Can you work these out from the model? Positions are in its coordinate system, mm. Face numbers are marked on the shaded views. A direction names the side the tool comes from. Round coordinates to 2 decimals unless told otherwise and drop trailing zeros. Loops run counter-clockwise (first coordinate to the right, second up) from the corner with the lowest first, then second, coordinate; pieces in that order, holes last. Notation, with made-up numbers: (64, 55.25) -> (84, 55.25) arc R9 ccw to (84, 61.25) -> close; hole circle Ø3 at (7, 1). An arc over 180 degrees is marked (long way). Use a Markdown table: item, result.
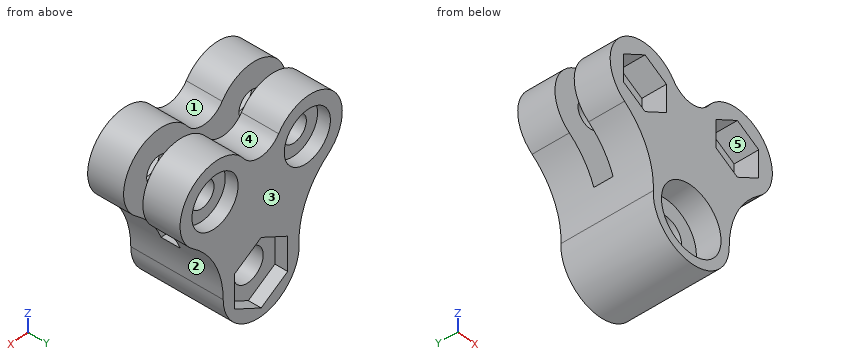
from build123d import *

# Parameters (mm, degrees)
SKETCH1_R           = 3.2639
SKETCH1_R_2         = 4.1021
BOSS_EXTRUDE1_DEPTH = 22.86
CUT_EXTRUDE1_DEPTH  = 4.7625
SKETCH3_R           = 8.1915
BOTTOM_CUTS_DEPTH   = 6.096
SKETCH4_R           = 6.35
TOP_CUTS_DEPTH      = 3.175


with BuildPart() as part:
    # Sketch1 → Boss-Extrude1 (new body)
    with BuildSketch(Plane(origin=(0, 0, 0), x_dir=(1, 0, 0), z_dir=(0, 1, 0))):
        with BuildLine():
            ThreePointArc((-10.440306098, 157.003610008), (-12.313301142, 147.763224627), (-18.350908637, 140.521668981))
            ThreePointArc((-18.350908637, 140.521668981), (-19.427506678, 125.875984036), (-4.807172888, 127.254748239))
            ThreePointArc((-4.807172888, 127.254748239), (0, 129.766974532), (4.807172888, 127.254748239))
            ThreePointArc((4.807172888, 127.254748239), (19.257850316, 125.71380556), (18.723788674, 140.236593192))
            ThreePointArc((18.723788674, 140.236593192), (12.626773217, 147.928609691), (10.4521, 157.49999996))
            ThreePointArc((10.4521, 157.49999996), (-0.24826502, 167.949151069), (-10.440306098, 157.003610008))
        make_face()
        with Locations((-12.7, 132.743860498)):
            Circle(SKETCH1_R, mode=Mode.SUBTRACT)
        with Locations((12.7, 132.743860498)):
            Circle(SKETCH1_R, mode=Mode.SUBTRACT)
        with Locations((0, 157.49999996)):
            Circle(SKETCH1_R_2, mode=Mode.SUBTRACT)
    extrude(amount=BOSS_EXTRUDE1_DEPTH)

    # Sketch2 → Cut-Extrude1 (cut)
    with BuildSketch(Plane(origin=(0, 8.89, 0), x_dir=(-1, 0, 0), z_dir=(0, -1, 0))):
        with BuildLine():
            ThreePointArc((-18.723788674, 140.236593192), (-19.257850316, 125.71380556), (-4.807172888, 127.254748239))
            ThreePointArc((-4.807172888, 127.254748239), (0, 129.766974532), (4.807172888, 127.254748239))
            ThreePointArc((4.807172888, 127.254748239), (19.427506678, 125.875984036), (18.350908637, 140.521668981))
            ThreePointArc((18.350908637, 140.521668981), (14.325271112, 144.466825655), (11.615435011, 149.40917398))
            ThreePointArc((11.615435011, 149.40917398), (-0.19007082, 149.859879464), (-11.994395391, 149.379229076))
            ThreePointArc((-11.994395391, 149.379229076), (-14.763447186, 144.369489602), (-18.723788674, 140.236593192))
        make_face()
    extrude(amount=-CUT_EXTRUDE1_DEPTH, mode=Mode.SUBTRACT)

    # Sketch3 → bottom-cuts (cut)
    with BuildSketch(Plane.XZ):
        with Locations((0, -157.49999996)):
            Circle(SKETCH3_R)
        Polygon((-18.57375, -129.352649355), (-18.57375, -136.135071642), (-12.7, -139.526282786), (-6.82625, -136.135071642), (-6.82625, -129.352649355), (-12.7, -125.961438211), align=None)
        Polygon((12.7, -125.961438211), (18.57375, -129.352649355), (18.57375, -136.135071642), (12.7, -139.526282786), (6.82625, -136.135071642), (6.82625, -129.352649355), align=None)
    extrude(amount=-BOTTOM_CUTS_DEPTH, mode=Mode.SUBTRACT)

    # Sketch4 → top-cuts (cut)
    with BuildSketch(Plane(origin=(0, 22.86, 0), x_dir=(1, 0, 0), z_dir=(0, 1, 0))):
        with Locations((-12.7, 132.743860498)):
            Circle(SKETCH4_R)
        with Locations((12.7, 132.743860498)):
            Circle(SKETCH4_R)
        Polygon((7.3025, 161.716100301), (0, 165.932200642), (-7.3025, 161.716100301), (-7.3025, 153.283899619), (0, 149.067799278), (7.3025, 153.283899619), align=None)
    extrude(amount=-TOP_CUTS_DEPTH, mode=Mode.SUBTRACT)


solid = part.part
1. I need wall thicknesses on line 1 (Z direction, x = 0, y = 4.5); line 2 (Y direction, x = 1, z = -135); line 3 (X direction, y = 6, z = -135). Which ranges of each line are inside material? Lowest first, please.
Answer sheet:
| item | result |
|---|---|
| line 1 | z = -167.95 to -165.69, -149.31 to -129.77 |
| line 2 | y = 0 to 8.89, 13.65 to 22.86 |
| line 3 | x = -22.05 to -18.57, -6.83 to 6.83, 18.57 to 22.05 |
2. Which directions (+Z, -Z, +X, -X, +Y, -Y) give clear straight access to the entire face, cutting with the end or side of a thin tool? Please do the marked faces 4 and 5.
Answer sheet:
| item | result |
|---|---|
| face 4 | +Z, +Y, -Y |
| face 5 | -Y |
3. I want a section at B-B (z = -160.5). Please give me the cut outline in (x, y) (1 decimal), plus the area to 3 significant figures.
Answer sheet:
| item | result |
|---|---|
| outline | (-10, 0) -> (-7.6, 0) -> (-7.6, 6.1) -> (-2.8, 6.1) -> (-2.8, 19.7) -> (-7.3, 19.7) -> (-7.3, 22.9) -> (-10, 22.9) -> close; (2.8, 6.1) -> (7.6, 6.1) -> (7.6, 0) -> (10, 0) -> (10, 22.9) -> (7.3, 22.9) -> (7.3, 19.7) -> (2.8, 19.7) -> close |
| area | 242 mm² |
4. If we mould it in two halves opening along X, with no side actions, what happens to the marked faces 1, 2 and 3? For each: +X half, -X half, draft (parallel to the pull), parting line (faces both ways), or undercut.
Answer sheet:
| item | result |
|---|---|
| face 1 | undercut |
| face 2 | +X half |
| face 3 | draft |
5. I want a section at A-A (x = -17). Please give me the cut outline in (y, z) (1 decimal), plus the area to 3 significant figures.
Answer sheet:
| item | result |
|---|---|
| outline | (0, -141.6) -> (8.9, -141.6) -> (8.9, -124.1) -> (0, -124.1) -> (0, -128.4) -> (6.1, -128.4) -> (6.1, -137) -> (0, -137) -> close; (13.7, -141.6) -> (22.9, -141.6) -> (22.9, -137.4) -> (19.7, -137.4) -> (19.7, -128.1) -> (22.9, -128.1) -> (22.9, -124.1) -> (13.7, -124.1) -> close |
| area | 234 mm² |
6. I want a section at C-C (y = 8). Please give me the cut outline in (x, z).
Answer sheet:
| item | result |
|---|---|
| outline | (-18.35, -140.52) arc R19.24 cw to (-10.44, -157) arc R10.45 ccw (long way) to (10.45, -157.5) arc R22.15 cw to (18.72, -140.24) arc R9.61 ccw (long way) to (4.81, -127.25) arc R5.86 cw to (-4.81, -127.25) arc R9.61 ccw (long way) to start; hole circle Ø6.53 at (-12.7, -132.74); hole circle Ø8.2 at (0, -157.5); hole circle Ø6.53 at (12.7, -132.74) |
7. I want a section at D-D (x = 2.5). Please give me the cut outline in (y, z) (1 decimal), plus the area to 3 significant figures.
Answer sheet:
| item | result |
|---|---|
| outline | (0, -167.6) -> (22.9, -167.6) -> (22.9, -164.5) -> (19.7, -164.5) -> (19.7, -160.8) -> (6.1, -160.8) -> (6.1, -165.3) -> (0, -165.3) -> close; (0, -149.7) -> (6.1, -149.7) -> (6.1, -154.2) -> (19.7, -154.2) -> (19.7, -150.5) -> (22.9, -150.5) -> (22.9, -129.2) -> (13.7, -129.2) -> (13.7, -149.8) -> (8.9, -149.8) -> (8.9, -129.2) -> (0, -129.2) -> close |
| area | 553 mm² |
8. Will these pins go through, and if not, where does the flat tip stop? pin 1 Ø6.5 at (x, z) = (-11.5, -135) entering from +Y (3 decimals); pin 2 Ø4 at (x, z) = (-12.7, -132.74) entering from +Y; pin 3 Ø1 at (y, z) = (15.5, -149) entering from -X; pin 4 Ø1.5 at (x, y) = (-3.5, 4) entering from -Z.
Answer sheet:
| item | result |
|---|---|
| pin 1 | stops at y = 19.685 |
| pin 2 | passes through |
| pin 3 | stops at x = -11.98 |
| pin 4 | stops at z = -167.58 |
